```python
from build123d import *

# Parameters (mm, degrees)
F0_W     = 76.2404734269
F0_H     = 59.8093401641
F1_DEPTH = 9.525
F2_W     = 8.5795149207
F2_H     = 75.9475912213
F3_DEPTH = 59.436
F4_W     = 389.8571208119
F4_H     = 18.9275667071
F5_DEPTH = 59.182
F7_D     = 22.225
F7_DEPTH = 9.526


with BuildPart() as f1:
    # F0 (on Top) → F1 (new body)
    with BuildSketch(Plane.XY):
        with Locations((24.8636114411, -6.689065136)):
            Rectangle(F0_W, F0_H)
    extrude(amount=-F1_DEPTH)

    # F2 (on face) → F3 (join)
    with BuildSketch(Plane.XZ.offset(36.593735218)):
        with Locations((58.6940906942, -47.4987956107)):
            Rectangle(F2_W, F2_H)
    extrude(amount=-F3_DEPTH)

    # F4 (on face) → F5 (join)
    with BuildSketch(Plane.XZ.offset(36.593735218)):
        with Locations((-131.9447122514, -94.9363745749)):
            Rectangle(F4_W, F4_H)
    extrude(amount=-F5_DEPTH)

    # F7 (through all, one way)
    with BuildSketch(Plane(origin=(0, 0, -9.525), x_dir=(1, 0, 0), z_dir=(0, 0, -1))):
        with Locations((26.1457208544, 7.0796483196)):
            Circle(F7_D / 2)
    extrude(amount=-F7_DEPTH, mode=Mode.SUBTRACT)


solid = f1.part
```
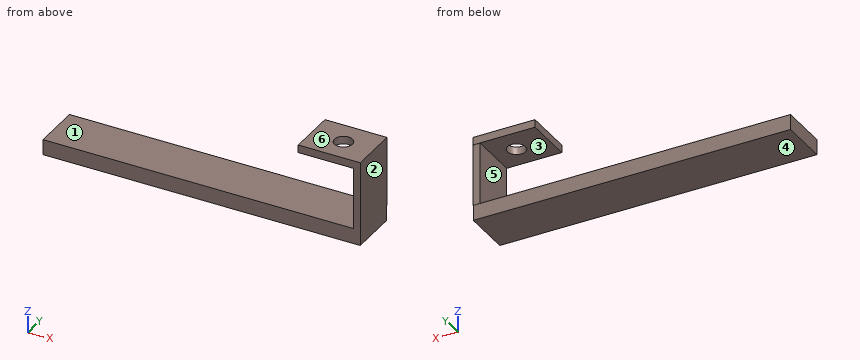
Source: CAD feature listing. Evaluate the final solid. Frame: model axes, mm. Face numbers are marked on the shaded views. A direction names the side the tool comes from. Give positions to 0.01 mm unless a question says otherwise; leave off trailing zeros. Write each loop counter-clockwise with the first axis right and the second up, starting at its lowest first coordinate (ties: lowest second). Pieces come first, ordered by that corner, then holes.
1. Section query A-A (y = -1.5). Return the cut outline in (x, z) (3 decimals).
2. Section query C-C (z = -40). Return the cut outline in (x, y).
3. First-contact query: pin 1 (2.5 mm diameter, centred on x = 57.5, z = -31, fed in from +Y); pin 2 (8 mm diameter, centred on y = -19.5, z = -54, fed in from -X); pin 3 (5 mm diameter, centred on x = -253, y = -20.5, fed in from +Z). Flat tips, straight axial feed; report the tip coordinate or a pass-through.
4. Section query D-D (x = -232). Return the cut outline in (y, z), then the cut area to 3 significant figures.
5. Section query B-B (y = -28). Return the cut outline in (x, z) (3 decimals).
6. Access query for the marked faces 1 and 2. Directions: +Z, -Z, +X, -X, +Y, -Y. A direction counts if a zero-diameter tool reaches every point of the face in a straight line with its end or side. Return the directions, or none.
7. Pull-direction query (Z, two-part tool) for the marked faces 3, 4, 5 and 6; classes: +Z half, -Z half, draft (parallel to the pull), parting line (faces both ways), or undercut.
8. Material intervals for line 1 along Z through (x, y) = (8, -11) (3 decimals); line 2 along Y through (x, z) = (-78, -87.5); line 3 along X through (y, z) = (-10.5, -39), sorted ascending.
Output values:
1. outline: (-326.873, -104.4) - (62.984, -104.4) - (62.984, 0) - (35.756, 0) - (35.756, -9.525) - (54.404, -9.525) - (54.404, -85.473) - (-326.873, -85.473) - close; (-13.257, -9.525) - (16.536, -9.525) - (16.536, 0) - (-13.257, 0) - close
2. outline: (54.4, -36.59) - (62.98, -36.59) - (62.98, 22.84) - (54.4, 22.84) - close
3. pin 1: stops at y = 22.84
3. pin 2: stops at x = 54.4
3. pin 3: stops at z = -85.47
4. outline: (-36.59, -104.4) - (22.59, -104.4) - (22.59, -85.47) - (-36.59, -85.47) - close
4. area: 1,120 mm2
5. outline: (-326.873, -104.4) - (62.984, -104.4) - (62.984, 0) - (-13.257, 0) - (-13.257, -9.525) - (54.404, -9.525) - (54.404, -85.473) - (-326.873, -85.473) - close
6. face 1: -X, +Y, -Y
6. face 2: +Z, -Z, +X, +Y, -Y
7. face 3: undercut
7. face 4: -Z half
7. face 5: undercut
7. face 6: +Z half
8. line 1: z = -104.4 to -85.473, -9.525 to 0
8. line 2: y = -36.59 to 22.59
8. line 3: x = 54.4 to 62.98
